```python
from build123d import *

# Parameters (mm, degrees)
PAD002_DEPTH            = 1
SKETCH007_R             = 1.4
SKETCH007_W             = 6
SKETCH007_H             = 8
PAD003_DEPTH            = 4
SKETCH013_W             = 2
SKETCH013_H             = 3.75
SKETCH013_H_2           = 5
PAD004_DEPTH            = 5
SKETCH014_W             = 41
SKETCH014_H             = 11.648772
SKETCH014_H_2           = 8.5
POCKET004_DEPTH         = 5.001
BODY001_PLACEMENT_ANGLE = 180


with BuildPart() as part:
    # Sketch006 → Pad002 (new body)
    with BuildSketch(Plane.XY):
        with BuildLine():
            Line((0.5, 0), (56.5, 0))
            ThreePointArc((56.5, 0), (56.853553, 0.146447), (57, 0.5))
            Line((57, 0.5), (57, 22.5))
            ThreePointArc((57, 22.5), (56.853553, 22.853553), (56.5, 23))
            Line((56.5, 23), (0.5, 23))
            ThreePointArc((0.5, 23), (0.146447, 22.853553), (0, 22.5))
            Line((0, 22.5), (0, 0.5))
            ThreePointArc((0, 0.5), (0.146447, 0.146447), (0.5, 0))
        make_face()
    extrude(amount=PAD002_DEPTH)

    # Sketch007 → Pad003 (join)
    with BuildSketch(Plane.XY):
        with Locations((3, 19.25)):
            Circle(SKETCH007_R)
        with Locations((3, 3.75)):
            Circle(SKETCH007_R)
        with Locations((54, 19.25)):
            Circle(SKETCH007_R)
        with Locations((54, 3.75)):
            Circle(SKETCH007_R)
        with Locations((3, 11.5)):
            Rectangle(SKETCH007_W, SKETCH007_H)
    extrude(amount=PAD003_DEPTH)

    # Sketch013 → Pad004 (join)
    with BuildSketch(Plane.XY):
        with Locations((7.1, 17.375)):
            Rectangle(SKETCH013_W, SKETCH013_H)
        with Locations((7.1, 5.625)):
            Rectangle(SKETCH013_W, SKETCH013_H)
        with Locations((50, 11.5)):
            Rectangle(SKETCH013_W, SKETCH013_H_2)
    extrude(amount=PAD004_DEPTH)

    # Sketch014 → Pocket004 (cut, through all)
    with BuildSketch(Plane.XY):
        with Locations((28.5, 20.324386)):
            Rectangle(SKETCH014_W, SKETCH014_H)
        with Locations((28.5, 4.25)):
            Rectangle(SKETCH014_W, SKETCH014_H_2)
    extrude(amount=POCKET004_DEPTH, mode=Mode.SUBTRACT)


with BuildPart() as part_1:
    # Body001 placement: moved
    add(part.part.moved(Location((0, 23, 16))).rotate(Axis((0, 23, 16), (-1, 0, 0)), BODY001_PLACEMENT_ANGLE))


solid = part_1.part
```
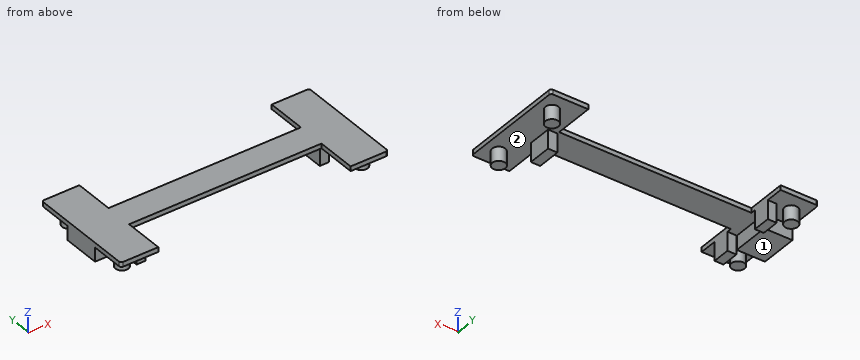
For this review, take the finished solid that the model builds, in its own axes (mm). Face numbers are marked on the shaded views. Coordinates: 2 decimals unless noted, no trailing zeros. Order: outer loops, then holes, each group sorted by start corner. A loop starts at its lowest first (then second) coordinate and runs counter-clockwise, first axis right, second up. Notation, with made-up numbers: (38.25, 16) -> (79.25, 16) arc R17 cw to (79.25, 28) -> close; hole circle Ø11 at (-0.5, 22.25). An arc over 180 degrees is marked (long way). Use CSV: the item, a comma, the result in double quotes. Start each with the question number.
Item 1: Draft analysis for pull direction X (two halves, no side actions). For the marked faces 1 and 2, state which applies: pulls with the +X half, pulls with the -X half, needs draft (parallel to the pull), parting line crosses it, or undercut.
Item 2: Wall thickness on probe 1 along X at (y, z) = (12.25, 14.75); probe 2 along Y at (x, z) = (4, 13.4); probe 3 along X at (y, z) = (4, 14.9): over which ranges is each line inside the solid? List them lowest first.
Item 3: We need section A-A, the plane y = 7. Give the boundary of the cut face in (x, z), then the cut area to 3 significant figures.
Item 4: We need section C-C, the plane x = 54. Give the boundary of the cut face in (y, z).
Item 5: We need section D-D, the plane y = 21.75. Give the boundary of the cut face in (x, z).
Item 6: Insertion check: pin 1 (2 mm diameter, centred on y = 10.5, z = 13.5, fed in from -X); pin 2 (0.6 mm diameter, centred on x = 7, z = 12, fed in from -Y); pin 3 (1 mm diameter, centred on x = 46, y = 14.5, fed in from -Z); pin 4 (0.9 mm diameter, centred on x = 2, z = 13, fed in from -Y). Each pin has a flat end and moves straight along its axis. Give the tip position at first contact, or say it passes through.
Item 7: We need section B-B, the plane z = 11.5. Give the boundary of the cut face in (x, y), then the cut area to 4 significant figures.
Derived:
1,face 1,"needs draft"
1,face 2,"undercut"
2,probe 1,"x = 0 to 6, 49 to 51"
2,probe 2,"y = 2.77 to 4.73, 7.5 to 15.5, 18.27 to 20.23"
2,probe 3,"x = 1.62 to 4.38, 6.1 to 8, 52.62 to 55.38"
3,outline,"(0, 15) -> (6.1, 15) -> (6.1, 11) -> (8, 11) -> (8, 16) -> (0, 16) -> close; (49, 15) -> (57, 15) -> (57, 16) -> (49, 16) -> close"
3,area,"23.6 mm^2"
4,outline,"(0, 15) -> (2.35, 15) -> (2.35, 12) -> (5.15, 12) -> (5.15, 15) -> (17.85, 15) -> (17.85, 12) -> (20.65, 12) -> (20.65, 15) -> (23, 15) -> (23, 16) -> (0, 16) -> close"
5,outline,"(0, 15) -> (8, 15) -> (8, 16) -> (0, 16) -> close; (49, 15) -> (57, 15) -> (57, 16) -> (49, 16) -> close"
6,pin 1,"stops at x = 0"
6,pin 2,"stops at y = 3.75"
6,pin 3,"stops at z = 15"
6,pin 4,"stops at y = 2.46"
7,outline,"(6.1, 3.75) -> (8, 3.75) -> (8, 7.5) -> (6.1, 7.5) -> close; (6.1, 15.5) -> (8, 15.5) -> (8, 19.25) -> (6.1, 19.25) -> close; (49, 9) -> (51, 9) -> (51, 14) -> (49, 14) -> close"
7,area,"24.25 mm^2"
